CAD build for the part. Positions are in the model's coordinates, mm. A direction names the side the tool comes from. Coordinates: 2 decimals unless noted, no trailing zeros. Loops run counter-clockwise (first coordinate to the right, second up) from the corner with the lowest first, then second, coordinate; pieces in that order, holes last. Notation, with made-up numbers: (75, 27.25) - (88, 27.25) arc R19 cw to (88, 35.25) - close; hole circle Ø2 at (-27.5, -20.5). An arc over 180 degrees is marked (long way). Put each result on its own line as item: value.
Autodesk Inventor part; units mm, degrees
ref_plane "YZ Plane" through (0, 0, 0) normal (1, 0, 0) x (0, 1, 0)
ref_plane "XZ Plane" through (0, 0, 0) normal (0, 1, 0) x (-1, 0, 0)
ref_plane "XY Plane" through (0, 0, 0) normal (0, 0, 1) x (1, 0, 0)
sketch "Skizze1" plane through (0, 0, 0) normal (0, 0, 1) x (1, 0, 0)
  line L0 (0, 0) -> (-13, 0)
  line L1 (-13, 0) -> (-13, -50)
  line L2 (-13, -50) -> (-10, -50)
  line L3 (-10, -50) -> (-10, -3)
  line L4 (-10, -3) -> (0, -3)
  line L5 (0, -3) -> (0, 0)
  line L6 (-13, 0) -> (0, 0)
  line L7 (0, 10) -> (0, -60)
  line L8 (0, 0) -> (13, 0)
  line L9 (13, 0) -> (13, -50)
  line L10 (13, -50) -> (10, -50)
  line L11 (10, -50) -> (10, -3)
  line L12 (10, -3) -> (0, -3)
  line L13 (13, 0) -> (0, 0)
  dimension "d0" = 13
  dimension "d1" = 50
  dimension "d2" = 3
  dimension "d3" = 47
extrude "Extrusion1" add sketch "Skizze1" along normal mid plane 15
sketch "Skizze2" plane through (-13, -50, 7.5) normal (-1, 0, 0) x (0, 0, 1)
  line L0 (-15, 0) -> (-15, 50)
  line L1 (-15, 0) -> (0, 0)
  line L2 (-15, 50) -> (0, 50)
  line L3 (0, 50) -> (0, 7.5)
  line L4 (-7.5, 0) -> (-7.5, 0)
  line L5 (-15, 7.5) -> (-15, 50)
  arc A0 (-15, 7.5) -> (-7.5, 0) centre (-7.5, 7.5) ccw
  arc A1 (-7.5, 0) -> (0, 7.5) centre (-7.5, 7.5) ccw
  circle A2 centre (-7.5, 7.5) radius 4
  line L6 (-15, 50) -> (0, 50)
  line L7 (0, 50) -> (0, 0)
  line L8 (0, 0) -> (-15, 0)
  line L9 (-15, 0) -> (-15, 50)
  point P0 (-7.5, 50)
  point P1 (0, 7.5)
  point P2 (-7.5, 0)
  point P3 (-7.5, 0)
  point P4 (-7.5, 0)
  point P5 (-15, 7.5)
  dimension "d6" = 7.5
  dimension "d7" = 8
extrude "Extrusion2" cut sketch "Skizze2" against normal through all contours L0 A0 L1 | A1 L7 L1 | A2
sketch "Skizze3" plane through (-13, 0, 7.5) normal (0, 1, 0) x (1, 0, 0)
  circle A0 centre (13, 7.5) radius 5
  dimension "d10" = 10
extrude "Extrusion3" cut sketch "Skizze3" against normal through all
sketch "Skizze4" plane through (-13, 0, 7.5) normal (0, 1, 0) x (1, 0, 0)
  circle A0 centre (13, 7.5) radius 5
  circle A1 centre (13, 7.5) radius 5
  circle A2 centre (13, 7.5) radius 7.5
  dimension "d13" = 2.5
extrude "Extrusion4" add sketch "Skizze4" along normal blind 10
thread "Gewinde1"
properties part number "ustück" material "Stahl"
Q1. Wall check: L1, parallel to X at y = -17, z = 4.75; L2, parallel to Y at x = 10.9, z = 0; L3, parallel to X at y = 3.5, z = 0. Give the ranges that are in metal, low to high. Write a range as from..to.
Determined:
L1: -13..-10, 10..13
L2: -50..-46.5, -38.5..0
L3: -7.5..-5, 5..7.5
Q2. Mould opens along Y. For faces 4 (the flat face through (-2, -3, -5)), 5 (the cylindrical face through (11.479, -38.534, -0.521)), 6 (the flat face through (9, 0, 0)) say: +Y half, -Y half, draft (parallel to the pull), parting line (faces both ways), or undercut.
Determined:
face 4: -Y half
face 5: undercut
face 6: +Y half
Q3. Pin check, flat tips, straight feed: pin 1 Ø6 at (x, z) = (0, 0) entering from +Y; pin 2 Ø5 at (x, z) = (9.5, -3) entering from -Y. Stop position of each tip, or through.
Determined:
pin 1: through
pin 2: y = -49.98
Q4. Tool access for faces 1 (the cylindrical face through (-7.493, 4.93, 0.33)), 2 (the flat face through (-10, -27, 0)), 3 (the cylindrical face through (11, -50, 0)): list every direction of +Z, -Z, +X, -X, +Y, -Y with a clear straight run to the whole face (end or side of a thin tool).
Determined:
face 1: +Y
face 2: +Z, -Z, -Y
face 3: +X, -X, -Y
Q5. Slice it at D-D, the plane z = -6.25. Give the cut face in (x, y), then the cut area to 3 significant figures.
Determined:
outline: (-13, -46.65) - (-10, -46.65) - (-10, -3) - (10, -3) - (10, -46.65) - (13, -46.65) - (13, 0) - (4.15, 0) - (4.15, 10) - (-4.15, 10) - (-4.15, 0) - (-13, 0) - close
area: 423 mm2
Q6. Slice it at B-B, the plane z = 0. Give the cut face in (x, y), then the cut area to 3 significant figures.
Determined:
outline: (-13, -50) - (-10, -50) - (-10, -46.5) - (-13, -46.5) - close; (-13, -38.5) - (-10, -38.5) - (-10, -3) - (-5, -3) - (-5, 10) - (-7.5, 10) - (-7.5, 0) - (-13, 0) - close; (5, -3) - (10, -3) - (10, -38.5) - (13, -38.5) - (13, 0) - (7.5, 0) - (7.5, 10) - (5, 10) - close; (10, -50) - (13, -50) - (13, -46.5) - (10, -46.5) - close
area: 332 mm2
Q7. Slice it at A-A, the plane y = -29. Give the cut face in (x, z), then the cut area to 3 significant figures.
Determined:
outline: (-13, -7.5) - (-10, -7.5) - (-10, 7.5) - (-13, 7.5) - close; (10, -7.5) - (13, -7.5) - (13, 7.5) - (10, 7.5) - close
area: 90.0 mm2
Q8. Slice it at C-C, the plane x = 3.25. Give the cut face in (y, z), then the cut area to 3 significant figures.
Determined:
outline: (-3, -7.5) - (0, -7.5) - (0, -6.76) - (10, -6.76) - (10, -3.8) - (-3, -3.8) - close; (-3, 3.8) - (10, 3.8) - (10, 6.76) - (0, 6.76) - (0, 7.5) - (-3, 7.5) - close
area: 81.4 mm2
